The listing builds one solid part. Answer for the finished solid, in the listing's coordinates (mm). Coordinates: 2 decimals unless noted, no trailing zeros. Loops run counter-clockwise (first coordinate to the right, second up) from the corner with the lowest first, then second, coordinate; pieces in that order, holes last. Notation, with made-up numbers: (21, 41) - (39, 41) arc R12 cw to (39, 60) - close; hole circle Ø6 at (64.25, 44). An arc over 180 degrees is marked (long way). Return JSON: item names as keys, results as strings. Group by question number.
1. Section B-B (x = 39) is taken. Write down the section's boundary in (y, z), and give its area (3 significant figures).
2. Section A-A (z = 1.95) is taken. Write down the section's boundary in (x, y).
3. Each of these flat-tipped pins is pushed along its axis until it touches: P1, Ø0.9, axis at x = -47, z = 1, coming from the -Y side; P2, Ø1.5, axis at y = 3, z = 1.5, coming from the +X side. Where does it stop, or does it pass through?
4. Find the intervals of material crossed by line 1 along Y through (x, z) = (-36, 0.8); line 2 along X through (y, z) = (-7, 0.4), in increasing order.
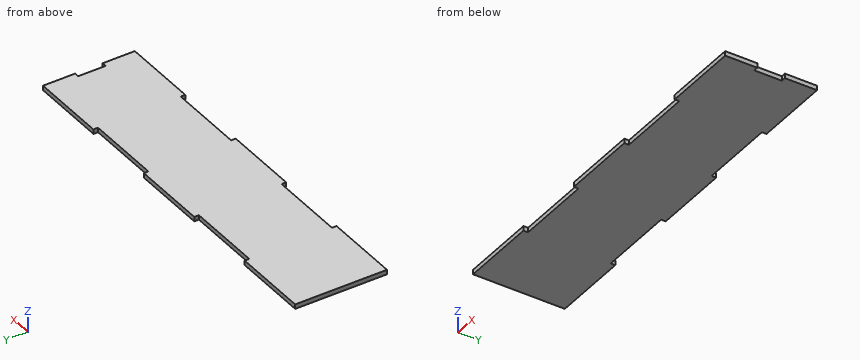
Autodesk Fusion 360 part; units mm, degrees
sketch "Sketch1" plane through (0, 0, 0) normal (0, 0, 1) x (1, 0, 0) in component "Step front"
  line L0 (125, 30) -> (-125, 30)
  line L1 (-125, 30) -> (-125, -30)
  line L2 (-125, -30) -> (125, -30)
  line L3 (125, -30) -> (125, 30)
  line L4 (125, 30) -> (-125, -30) construction
  line L5 (-125, 30) -> (125, -30) construction
  line L6 (-125, 30) -> (-75, 30)
  line L7 (-75, 30) -> (-75, 27)
  line L8 (-75, 27) -> (-125, 27)
  line L9 (-125, 27) -> (-125, 30)
  line L10 (-25, 27) -> (-75, 27)
  line L11 (-25, 30) -> (-25, 27)
  line L12 (-75, 30) -> (-25, 30)
  line L13 (-75, 30) -> (-75, -30)
  line L14 (25, 27) -> (-25, 27)
  line L15 (25, 30) -> (25, 27)
  line L16 (-25, 30) -> (25, 30)
  line L17 (-25, 30) -> (-25, -30)
  line L18 (75, 27) -> (25, 27)
  line L19 (75, 30) -> (75, 27)
  line L20 (25, 30) -> (75, 30)
  line L21 (25, 30) -> (25, -30)
  line L22 (125, 27) -> (75, 27)
  line L23 (125, 30) -> (125, 27)
  line L24 (75, 30) -> (125, 30)
  line L25 (75, 30) -> (75, -30)
  line L26 (-75, -30) -> (-125, -30)
  line L27 (-75, -27) -> (-75, -30)
  line L28 (-125, -27) -> (-75, -27)
  line L29 (-125, -27) -> (-125, -30)
  line L30 (-25, -30) -> (-75, -30)
  line L31 (-25, -27) -> (-25, -30)
  line L32 (-75, -27) -> (-25, -27)
  line L33 (-75, -27) -> (-75, -30)
  line L34 (25, -30) -> (-25, -30)
  line L35 (25, -27) -> (25, -30)
  line L36 (-25, -27) -> (25, -27)
  line L37 (-25, -27) -> (-25, -30)
  line L38 (75, -30) -> (25, -30)
  line L39 (75, -27) -> (75, -30)
  line L40 (25, -27) -> (75, -27)
  line L41 (25, -27) -> (25, -30)
  line L42 (125, -30) -> (75, -30)
  line L43 (125, -27) -> (125, -30)
  line L44 (75, -27) -> (125, -27)
  line L45 (75, -27) -> (75, -30)
  dimension "d1" = 250
  dimension "d2" = 60
  dimension "d9" = 50
  dimension "d10" = 3
extrude "Extrude3" add sketch "Sketch1" along normal blind 3 contours L0 L3 L19 L22 L23 L24 L25 | L3 L22 L25 L44 | L0 L11 L14 L15 L16 L17 L21 | L18 L21 L25 L40 | L2 L3 L25 L39 L42 L43 L44 L45 | L14 L17 L21 L36 | L0 L1 L6 L7 L8 L9 L13 | L10 L13 L17 L32 | L2 L17 L21 L31 L34 L35 L36 L37 L41 | L1 L8 L13 L28 | L1 L2 L13 L26 L27 L28 L29 L33 in component "Step front"
sketch "Sketch3" plane through (0, 0, 3) normal (0, 0, 1) x (-1, 0, 0) in component "Step front"
  line L0 (-25, 27) -> (-75, 27)
  line L1 (-75, 27) -> (-75, 30)
  line L2 (-75, 30) -> (-125, 30)
  line L3 (-125, 30) -> (-125, -30)
  line L4 (-125, -30) -> (-75, -30)
  line L5 (-75, -30) -> (-75, -27)
  line L6 (-75, -27) -> (-25, -27)
  line L7 (-25, -27) -> (-25, -30)
  line L8 (-25, -30) -> (25, -30)
  line L9 (25, -30) -> (25, -27)
  line L10 (25, -27) -> (75, -27)
  line L11 (75, -27) -> (75, -30)
  line L12 (75, -30) -> (125, -30)
  line L13 (125, -30) -> (125, 30)
  line L14 (125, 30) -> (75, 30)
  line L15 (75, 30) -> (75, 27)
  line L16 (75, 27) -> (25, 27)
  line L17 (25, 27) -> (25, 30)
  line L18 (25, 30) -> (-25, 30)
  line L19 (-25, 30) -> (-25, 27)
  line L20 (-125, -30) -> (-122, -30) construction
  line L21 (-122, -30) -> (-122, -8) construction
  line L22 (-122, -8) -> (-125, -8) construction
  line L23 (-125, -8) -> (-125, -30) construction
  line L24 (-125, 30) -> (-122, 30) construction
  line L25 (-122, 30) -> (-122, 8) construction
  line L26 (-122, 8) -> (-125, 8) construction
  line L27 (-125, 8) -> (-125, 30) construction
  line L28 (-125, -9) -> (-122, -9)
  line L29 (-122, -9) -> (-122, 9)
  line L30 (-122, 9) -> (-125, 9)
  line L31 (-125, 9) -> (-125, -9)
  dimension "d17" = 22
  dimension "d18" = 3
  dimension "d19" = 22
extrude "Extrude4" cut sketch "Sketch3" against normal blind 12 contours L3 L28 L29 L30 L31 in component "Step front"
sketch "Sketch1 (2)" plane through (0, 0, 3) normal (0, 0, 1) x (-1, 0, 0)
  line L0 (-122, -9) -> (-125, -9)
  line L1 (-125, -9) -> (-125, -30)
  line L2 (-125, -30) -> (-75, -30)
  line L3 (-75, -30) -> (-75, -27)
  line L4 (-75, -27) -> (-25, -27)
  line L5 (-25, -27) -> (-25, -30)
  line L6 (-25, -30) -> (25, -30)
  line L7 (25, -30) -> (25, -27)
  line L8 (25, -27) -> (75, -27)
  line L9 (75, -27) -> (75, -30)
  line L10 (75, -30) -> (125, -30)
  line L11 (125, -30) -> (125, 30)
  line L12 (125, 30) -> (75, 30)
  line L13 (75, 30) -> (75, 27)
  line L14 (75, 27) -> (25, 27)
  line L15 (25, 27) -> (25, 30)
  line L16 (25, 30) -> (-25, 30)
  line L17 (-25, 30) -> (-25, 27)
  line L18 (-25, 27) -> (-75, 27)
  line L19 (-75, 27) -> (-75, 30)
  line L20 (-75, 30) -> (-125, 30)
  line L21 (-125, 30) -> (-125, 9)
  line L22 (-125, 9) -> (-122, 9)
  line L23 (-122, 9) -> (-122, -9)
component "Step front" placed x (1, 0, 0) y (0, 1, 0) z (0, 0, 1) at (0, 0, 0)
The answers:
{
 "1": {"outline": "(-27, 0) - (27, 0) - (27, 3) - (-27, 3) - close", "area": "162 mm2"},
 "2": {"outline": "(-125, -30) - (-75, -30) - (-75, -27) - (-25, -27) - (-25, -30) - (25, -30) - (25, -27) - (75, -27) - (75, -30) - (125, -30) - (125, -9) - (122, -9) - (122, 9) - (125, 9) - (125, 30) - (75, 30) - (75, 27) - (25, 27) - (25, 30) - (-25, 30) - (-25, 27) - (-75, 27) - (-75, 30) - (-125, 30) - close"},
 "3": {"P1": "stops at y = -27", "P2": "stops at x = 122"},
 "4": {"line 1": "y = -27 to 27", "line 2": "x = -125 to 122"}
}
